Design review of the part built by this model. Coordinates are the model's own, in mm. A direction names the side the tool comes from. Give positions to 0.01 mm unless a question says otherwise; leave off trailing zeros. Loops run counter-clockwise (first coordinate to the right, second up) from the corner with the lowest first, then second, coordinate; pieces in that order, holes last. Notation, with made-up numbers: M -36,57.5 L 7,57.5 A27 ccw 7,87.5 Z; hole C 56.5,-29 d2. An arc over 180 degrees is marked long. Answer as CSV lines item,"result".
```python
from build123d import *

# Parameters (mm, degrees)
F0_W          = 120
F0_H          = 180
F1_DEPTH      = 30
F2_W          = 65
F2_H          = 50
F4_DEPTH      = 50
F3_W          = 65
F3_H          = 50
F5_DEPTH      = 50
F6_R          = 3
F7_R          = 2.5
F8_DEPTH      = 25
F8_DEPTH_BACK = 25


with BuildPart() as f1:
    # F0 (on Top) → F1 (new body, symmetric)
    with BuildSketch(Plane.XY):
        Rectangle(F0_W, F0_H)
    extrude(amount=F1_DEPTH, both=True)

    # F2 (on face) → F4 (cut)
    with BuildSketch(Plane.YZ.offset(60)):
        with Locations((-47.5, 5)):
            Rectangle(F2_W, F2_H)
        with Locations((47.5, 5)):
            Rectangle(F2_W, F2_H)
    extrude(amount=-F4_DEPTH, mode=Mode.SUBTRACT)

    # F3 (on face) → F5 (cut)
    with BuildSketch(Plane(origin=(-60, 0, 0), x_dir=(0, -1, 0), z_dir=(-1, 0, 0))):
        with Locations((-47.5, 5)):
            Rectangle(F3_W, F3_H)
        with Locations((47.5, 5)):
            Rectangle(F3_W, F3_H)
    extrude(amount=-F5_DEPTH, mode=Mode.SUBTRACT)

    # F6
    f6_edges = [f1.edges().sort_by_distance(p)[0] for p in [
        (0, -90, 30),
        (0, 90, 30),
        (0, -90, -30),
        (0, 90, -30),
    ]]
    fillet(f6_edges, radius=F6_R)

    # F7 (on face) → F8 (cut, two sides)
    with BuildSketch(Plane.XY.offset(-20)) as f8_sk:
        with Locations((50, -65)):
            Circle(F7_R)
        with Locations((50, -25)):
            Circle(F7_R)
        with Locations((20, -65)):
            Circle(F7_R)
        with Locations((20, -25)):
            Circle(F7_R)
        with Locations((48.7637452036, 25)):
            Circle(F7_R)
        with Locations((18.7637452036, 25)):
            Circle(F7_R)
        with Locations((18.7637452036, 65)):
            Circle(F7_R)
        with Locations((48.7637452036, 65)):
            Circle(F7_R)
    extrude(amount=-F8_DEPTH, mode=Mode.SUBTRACT)
    extrude(f8_sk.sketch, amount=F8_DEPTH_BACK, mode=Mode.SUBTRACT)


solid = f1.part
```
1. We need section C-C, the plane z = 23.5. Write out the cut boundary in (x, y), plus the area to 3 significant figures.
Answer block:
outline,"M -60,-90 L 60,-90 L 60,-80 L 10,-80 L 10,-15 L 60,-15 L 60,15 L 10,15 L 10,80 L 60,80 L 60,90 L -60,90 L -60,80 L -10,80 L -10,15 L -60,15 L -60,-15 L -10,-15 L -10,-80 L -60,-80 Z"
area,"8,600 mm²"
2. We need section D-D, the plane y = 72.5. Write out the cut boundary in (x, z), plus the area to 3 significant figures.
Answer block:
outline,"M -60,-30 L 60,-30 L 60,-20 L 10,-20 L 10,30 L -10,30 L -10,-20 L -60,-20 Z"
area,"2,200 mm²"
3. For P1, Ø25, axis at y = -46, z = -6.5, coming from the +X side; P2, Ø3, axis at x = 50, y = -65, coming from the +Z side; P3, Ø3, axis at y = -53.5, z = 5, coming from the -X side; P4, Ø25, axis at x = 38, y = -55.5, coming from the +Z side, all flat-tipped, find the tip position at first contact; note any pin that passes through.
Answer block:
P1,"x = 10"
P2,"through"
P3,"x = -10"
P4,"z = -20"
4. For faces 4 (the flat face through (35, 15, 5)), 5 (the flat face through (-35, 48, -20)), 6 (the flat face through (-1, 1, -30)), list the 3-axis set-ups (+Z, -Z, +X, -X, +Y, -Y) from which the entire face can be reached by the end or side of a thin tool; tool diameter is ignored.
Answer block:
face 4,"+Z, +X"
face 5,"+Z, -X"
face 6,"-Z, +X, -X, +Y, -Y"
5. We need section B-B, the plane y = 25. Write out the cut boundary in (x, z).
Answer block:
outline,"M -60,-30 L 16.26,-30 L 16.26,-20 L 10,-20 L 10,30 L -10,30 L -10,-20 L -60,-20 Z; M 21.26,-30 L 46.26,-30 L 46.26,-20 L 21.26,-20 Z; M 51.26,-30 L 60,-30 L 60,-20 L 51.26,-20 Z"
6. We need section A-A, the plane x = -38. Write out the cut boundary in (y, z), plus the area to 3 significant figures.
Answer block:
outline,"M -90,-27 A3 ccw -87,-30 L 87,-30 A3 ccw 90,-27 L 90,27 A3 ccw 87,30 L 80,30 L 80,-20 L 15,-20 L 15,30 L -15,30 L -15,-20 L -80,-20 L -80,30 L -87,30 A3 ccw -90,27 Z"
area,"4,290 mm²"
7. To check wall thickness, follow L1, parallel to Y at x = -26, z = -8.5; L2, parallel to Y at x = 20, z = -26; L3, parallel to Z at x = -53.5, y = -78. State the ranges of each line that lie inside material, in increasing order. Write a range as [from, to].
Answer block:
L1,"[-90, -80], [-15, 15], [80, 90]"
L2,"[-90, -67.5], [-62.5, -27.5], [-22.5, 22.83], [27.17, 62.83], [67.17, 90]"
L3,"[-30, -20]"
8. The part is to be moulded in two halves that separate along X. For faces 1 (the cylindrical face through (18.44, 27.48, -24.93)), 2 (the flat face through (-60, -7, -7)), 3 (the flat face through (-35, -80, 5)), say which applies: pulls with the +X half, pulls with the -X half, needs draft (parallel to the pull), parting line crosses it, or undercut.
Answer block:
face 1,"undercut"
face 2,"pulls with the -X half"
face 3,"needs draft"
